```python
from build123d import *

# Parameters (mm, degrees)
SKETCH_1_W          = 46
SKETCH_1_H          = 56
EXTRUDE_1_DEPTH     = 2.5
FILLET_1_R          = 6
SKETCH_2_R          = 1.5
CUT_EXTRUDE_1_DEPTH = 10
SKETCH_3_R          = 3
CUT_EXTRUDE_2_DEPTH = 10


with BuildPart() as part:
    # 草图1 → 凸台-拉伸1 (new body)
    with BuildSketch(Plane.XY):
        Rectangle(SKETCH_1_W, SKETCH_1_H)
    extrude(amount=EXTRUDE_1_DEPTH)

    # 圆角1
    fillet_1_edges = [part.edges().sort_by_distance(p)[0] for p in [
        (23, -28, 1.25),
        (-23, -28, 1.25),
        (-23, 28, 1.25),
        (23, 28, 1.25),
    ]]
    fillet(fillet_1_edges, radius=FILLET_1_R)

    # 草图2 → 切除-拉伸1 (cut)
    with BuildSketch(Plane.XY.offset(2.5)):
        with Locations((-19, 0)):
            Circle(SKETCH_2_R)
        with Locations((-7, 0)):
            Circle(SKETCH_2_R)
        with Locations((7, 0)):
            Circle(SKETCH_2_R)
        with Locations((19, 0)):
            Circle(SKETCH_2_R)
    extrude(amount=-CUT_EXTRUDE_1_DEPTH, mode=Mode.SUBTRACT)

    # 草图3 → 切除-拉伸2 (cut)
    with BuildSketch(Plane.XY.offset(2.5)):
        with Locations((-14, 7)):
            Circle(SKETCH_3_R)
        with Locations((0, 7)):
            Circle(SKETCH_3_R)
        with Locations((14, 7)):
            Circle(SKETCH_3_R)
        with Locations((-14, -7)):
            Circle(SKETCH_3_R)
        with Locations((0, -7)):
            Circle(SKETCH_3_R)
        with Locations((14, -7)):
            Circle(SKETCH_3_R)
        with Locations((-14, 21)):
            Circle(SKETCH_3_R)
        with Locations((0, 21)):
            Circle(SKETCH_3_R)
        with Locations((14, 21)):
            Circle(SKETCH_3_R)
        with Locations((14, -21)):
            Circle(SKETCH_3_R)
        with Locations((0, -21)):
            Circle(SKETCH_3_R)
        with Locations((-14, -21)):
            Circle(SKETCH_3_R)
    extrude(amount=-CUT_EXTRUDE_2_DEPTH, mode=Mode.SUBTRACT)


solid = part.part
```
Source: CAD feature listing. Evaluate the final solid. Frame: model axes, mm. Give positions to 0.01 mm unless a question says otherwise; leave off trailing zeros. Order: outer loops, then holes, each group sorted by start corner. A loop starts at its lowest first (then second) coordinate and runs counter-clockwise, first axis right, second up. Notation, with made-up numbers: (-37, 78) -> (7, 78) arc R12 ccw to (7, 84) -> close; hole circle Ø4 at (59, 18). An arc over 180 degrees is marked (long way). Use a Markdown table: item, result.
Q1. Section B-B (y = 0). Return the cut outline in (x, z), and give its area (3 significant figures).
A:
| item | result |
|---|---|
| outline | (-23, 0) -> (-20.5, 0) -> (-20.5, 2.5) -> (-23, 2.5) -> close; (-17.5, 0) -> (-8.5, 0) -> (-8.5, 2.5) -> (-17.5, 2.5) -> close; (-5.5, 0) -> (5.5, 0) -> (5.5, 2.5) -> (-5.5, 2.5) -> close; (8.5, 0) -> (17.5, 0) -> (17.5, 2.5) -> (8.5, 2.5) -> close; (20.5, 0) -> (23, 0) -> (23, 2.5) -> (20.5, 2.5) -> close |
| area | 85.0 mm^2 |
Q2. Pull-direction query (X, two-part tool) for faces 1 (the face through (0, 0, 2.5)), 2 (the face through (-0.65, 18.07, 1.27)), 3 (the face through (21.289, 26.196, 1.268)), 4 (the face through (-21.289, -26.196, 1.268)); classes: +X half, -X half, draft (parallel to the pull), parting line (faces both ways), or undercut.
A:
| item | result |
|---|---|
| face 1 | draft |
| face 2 | undercut |
| face 3 | +X half |
| face 4 | -X half |
Q3. Section C-C (y = -21). Return the cut outline in (x, z).
A:
| item | result |
|---|---|
| outline | (-23, 0) -> (-17, 0) -> (-17, 2.5) -> (-23, 2.5) -> close; (-11, 0) -> (-3, 0) -> (-3, 2.5) -> (-11, 2.5) -> close; (3, 0) -> (11, 0) -> (11, 2.5) -> (3, 2.5) -> close; (17, 0) -> (23, 0) -> (23, 2.5) -> (17, 2.5) -> close |
Q4. Section D-D (z = 1.05). State how many separate pieces and enclosed holes the cut face has, and give its area (3 significant figures).
A:
| item | result |
|---|---|
| separate pieces | 1 |
| enclosed holes | 16 |
| area | 2,180 mm^2 |
Q5. Section A-A (x = -14). Return the cut outline in (y, z), and give its area (3 significant figures).
A:
| item | result |
|---|---|
| outline | (-28, 0) -> (-24, 0) -> (-24, 2.5) -> (-28, 2.5) -> close; (-18, 0) -> (-10, 0) -> (-10, 2.5) -> (-18, 2.5) -> close; (-4, 0) -> (4, 0) -> (4, 2.5) -> (-4, 2.5) -> close; (10, 0) -> (18, 0) -> (18, 2.5) -> (10, 2.5) -> close; (24, 0) -> (28, 0) -> (28, 2.5) -> (24, 2.5) -> close |
| area | 80.0 mm^2 |
Q6. Material intervals for line 1 (Y direction, x = -14, z = 1.9); line 2 (X direction, y = -6.5, z = 1.15); line 3 (X direction, y = -8, z = 1.3), sorted ascending. Write a range as [from, to].
A:
| item | result |
|---|---|
| line 1 | [-28, -24], [-18, -10], [-4, 4], [10, 18], [24, 28] |
| line 2 | [-23, -16.96], [-11.04, -2.96], [2.96, 11.04], [16.96, 23] |
| line 3 | [-23, -16.83], [-11.17, -2.83], [2.83, 11.17], [16.83, 23] |
Q7. First-contact query: P1, Ø5, axis at x = 0, y = -7, coming from the +Z side. Flat tip, straight axial feed; report the tip coordinate or a pass-through.
A:
| item | result |
|---|---|
| P1 | through |
